from build123d import *

# Parameters (mm, degrees)
F0_W     = 37
F0_H     = 26.5
F1_DEPTH = 26
F2_W     = 34
F2_H     = 8
F2_R     = 3.738116
F3_DEPTH = 26.501
F4_W     = 20
F4_H     = 8
F5_DEPTH = 34
F7_DEPTH = 26.501


with BuildPart() as f1:
    # F0 (on Top) → F1 (new body)
    with BuildSketch(Plane.XY):
        with Locations((-10.29259, 13.25)):
            Rectangle(F0_W, F0_H)
    extrude(amount=-F1_DEPTH)

    # F2 (on Front) → F3 (cut, through all)
    with BuildSketch(Plane.XZ):
        with Locations((-11.79259, -17.5)):
            Rectangle(F2_W, F2_H)
        with Locations((-20.547456, -6.75)):
            Circle(F2_R)
        with Locations((-2.956501, -6.75)):
            Circle(F2_R)
    extrude(amount=-F3_DEPTH, mode=Mode.SUBTRACT)

    # F4 (on face) → F5 (cut)
    with BuildSketch(Plane.YZ.offset(8.20741)):
        with Locations((13.25, -7)):
            Rectangle(F4_W, F4_H)
    extrude(amount=-F5_DEPTH, mode=Mode.SUBTRACT)

    # F6 (on face) → F7 (cut, through all)
    with BuildSketch(Plane(origin=(0, 26.5, 0), x_dir=(-1, 0, 0), z_dir=(0, 1, 0))):
        Polygon((-8.20741, 0), (-8.20741, -3), (-5.20741, 0), align=None)
        Polygon((-8.20741, -23), (-8.20741, -26), (-5.20741, -26), align=None)
    extrude(amount=-F7_DEPTH, mode=Mode.SUBTRACT)


solid = f1.part
Geometry check sheet. Reference: the model listing, model coordinates, mm. A direction names the side the tool comes from. Coordinates: 2 decimals unless noted, no trailing zeros. Order: outer loops, then holes, each group sorted by start corner. A loop starts at its lowest first (then second) coordinate and runs counter-clockwise, first axis right, second up. Notation, with made-up numbers: (59, 38.25) -> (88, 38.25) arc R30 ccw to (88, 72.25) -> close; hole circle Ø9 at (-26.5, -26). An arc over 180 degrees is marked (long way). Use a Markdown table: item, result. Add a question column.
1. Cross-section at D-D (y = 6.5). Enter the section's corners in (x, z).
2. Set-up check for faces 1 (the face through (8.207, 13, -15)), 2 (the face through (-12, 13, -21.5)), 3 (the face through (-9, 13, -3)): record each of +Z, -Z, +X, -X, +Y, -Y from which the full face is reachable in a straight line by a thin tool's end or side.
3. Cross-section at C-C (y = 25). Enter the section's corners in (x, z).
4. Material ranges on L1, parallel to Z at x = -17, y = 14.5; L2, parallel to Y at x = -12.5, z = -10; L3, parallel to Z at x = 3, y = 25.25, recorded low to high.
5. Go/stop test with flat-tipped pins: pin 1 Ø9 at (y, z) = (17, -7.5) entering from +X; pin 2 Ø6.5 at (x, z) = (-2.96, -6.75) entering from -Y; pin 3 Ø4 at (y, z) = (17.5, -16.5) entering from -X. Record where each tip stops, or that it passes through.
6. Cross-section at A-A (x = -13.5). Enter the section's corners in (y, z).
7. Cross-section at B-B (z = -6.75). Enter the section's corners in (x, y).
8. Mould release check, pull along X, two halves, no side actions. Record for faces 4 (the face through (-17.1, 1.6, -8.2)), 5 (the face through (6.73, 13.44, -1.52)), 6 (the face through (-9, 23.25, -7)): pulls with the +X half, pulls with the -X half, needs draft (parallel to the pull), parting line crosses it, or undercut.
Filled sheet:
| question | item | result |
|---|---|---|
| 1 | outline | (-28.79, -26) -> (5.21, -26) -> (8.21, -23) -> (8.21, -11) -> (-25.79, -11) -> (-25.79, -3) -> (8.21, -3) -> (5.21, 0) -> (-28.79, 0) -> (-28.79, -13.5) -> (5.21, -13.5) -> (5.21, -21.5) -> (-28.79, -21.5) -> close |
| 2 | face 1 | +Z, -Z, +X, +Y, -Y |
| 2 | face 2 | -X, +Y, -Y |
| 2 | face 3 | +X |
| 3 | outline | (-28.79, -26) -> (5.21, -26) -> (8.21, -23) -> (8.21, -3) -> (5.21, 0) -> (-28.79, 0) -> (-28.79, -13.5) -> (5.21, -13.5) -> (5.21, -21.5) -> (-28.79, -21.5) -> close; hole circle Ø7.48 at (-20.55, -6.75); hole circle Ø7.48 at (-2.96, -6.75) |
| 4 | L1 | -26 to -21.5, -13.5 to -11, -3 to 0 |
| 4 | L2 | 0 to 3.25, 23.25 to 26.5 |
| 4 | L3 | -26 to -21.5, -13.5 to 0 |
| 5 | pin 1 | x = 8.21 |
| 5 | pin 2 | through |
| 5 | pin 3 | x = 5.21 |
| 6 | outline | (0, -26) -> (26.5, -26) -> (26.5, -21.5) -> (0, -21.5) -> close; (0, -13.5) -> (26.5, -13.5) -> (26.5, 0) -> (0, 0) -> close; hole (3.25, -11) -> (23.25, -11) -> (23.25, -3) -> (3.25, -3) -> close |
| 7 | outline | (-28.79, 0) -> (-24.29, 0) -> (-24.29, 3.25) -> (-25.79, 3.25) -> (-25.79, 23.25) -> (-24.29, 23.25) -> (-24.29, 26.5) -> (-28.79, 26.5) -> close; (-16.81, 0) -> (-6.69, 0) -> (-6.69, 3.25) -> (-16.81, 3.25) -> close; (-16.81, 23.25) -> (-6.69, 23.25) -> (-6.69, 26.5) -> (-16.81, 26.5) -> close; (0.78, 0) -> (8.21, 0) -> (8.21, 3.25) -> (0.78, 3.25) -> close; (0.78, 23.25) -> (8.21, 23.25) -> (8.21, 26.5) -> (0.78, 26.5) -> close |
| 8 | face 4 | undercut |
| 8 | face 5 | pulls with the +X half |
| 8 | face 6 | needs draft |
